Verification items for the finished model (mm, model axes). A direction names the side the tool comes from. Coordinates: 2 decimals unless noted, no trailing zeros. Loops run counter-clockwise (first coordinate to the right, second up) from the corner with the lowest first, then second, coordinate; pieces in that order, holes last. Notation, with made-up numbers: M 31,61.5 L 40,61.5 A10 cw 40,80.5 Z; hole C 58.25,23 d7. An arc over 180 degrees is marked long. Write item = value, one per line. Start each with the question number.
```python
from build123d import *

# Parameters (mm, degrees)
F3_DEPTH = 6.001
F4_R     = 1.5
F5_DEPTH = 3.5
F6_R     = 1.25
F7_DEPTH = 11.501


with BuildPart() as f1:
    # F0 (on Top) → F1 (revolve)
    with BuildSketch(Plane.XY):
        Polygon((3, -12), (3, -4.699), (1.5, -4.699), (0.23, -3.965765), (0.23, -4.295025), (-3, -6.159867), (-3, -12), align=None)
    revolve(axis=Axis((1.9254176877, 0, 0), (1, 0, 0)))

    # F2 (on face) → F3 (cut, through all)
    with BuildSketch(Plane.YZ.offset(3)):
        with BuildLine():
            ThreePointArc((11.313708499, 4), (9.0433383971, 7.8878406827), (5.5, 10.6653645039))
            Line((5.5, 10.6653645039), (5.5, 4))
            Line((5.5, 4), (11.313708499, 4))
        make_face()
        with BuildLine():
            Line((4.6723228698, -0.5), (11.9895788083, -0.5))
            ThreePointArc((11.9895788083, -0.5), (11.9973944192, -0.2500542947), (12, 0))
            ThreePointArc((12, 0), (11.9973944192, 0.2500542947), (11.9895788083, 0.5))
            Line((11.9895788083, 0.5), (4.6723228698, 0.5))
            ThreePointArc((4.6723228698, 0.5), (4.6923259779, 0.2503555818), (4.699, 0))
            ThreePointArc((4.699, 0), (4.6923259779, -0.2503555818), (4.6723228698, -0.5))
        make_face()
        with BuildLine():
            Line((-10, -0.5), (-4.6723228698, -0.5))
            ThreePointArc((-4.6723228698, -0.5), (-4.699, 0), (-4.6723228698, 0.5))
            Line((-4.6723228698, 0.5), (-10, 0.5))
            Line((-10, 0.5), (-10, -0.5))
        make_face()
        with BuildLine():
            Line((-4.6723228698, -0.5), (4.6723228698, -0.5))
            ThreePointArc((4.6723228698, -0.5), (4.6923259779, -0.2503555818), (4.699, 0))
            ThreePointArc((4.699, 0), (4.6923259779, 0.2503555818), (4.6723228698, 0.5))
            Line((4.6723228698, 0.5), (-4.6723228698, 0.5))
            ThreePointArc((-4.6723228698, 0.5), (-4.699, 0), (-4.6723228698, -0.5))
        make_face()
    extrude(amount=-F3_DEPTH, mode=Mode.SUBTRACT)

    # F4 (on face) → F5 (cut, through all)
    with BuildSketch(Plane.XY.offset(4)):
        with Locations((0, 8.5)):
            Circle(F4_R)
    extrude(amount=-F5_DEPTH, mode=Mode.SUBTRACT)

    # F6 (on face) → F7 (cut, through all)
    with BuildSketch(Plane.XY.offset(-0.5)):
        with Locations((0, 8.5)):
            Circle(F6_R)
    extrude(amount=-F7_DEPTH, mode=Mode.SUBTRACT)


solid = f1.part
```
Q1. Mould release check, pull along Y, two halves, no side actions. Record for faces 5 (the face through (0, 5.5, 7)), 6 (the face through (-0.27, 7.28, -4.97)), 7 (the face through (0, -8, -0.5)): +Y half, -Y half, draft (parallel to the pull), parting line (faces both ways), or undercut.
Q2. Sectioned sample at C-C on z = 0. Record the cut outline in (x, y).
Q3. Set-up check for faces 1 (the face through (1, 7, 4)), 2 (the face through (1.4, 8.8, -0.5)), 3 (the face through (-0.69, 0.101, 4.825)), 4 (the face through (0.43, 0.08, 4.08)): record each of +Z, -Z, +X, -X, +Y, -Y from which the full face is reachable in a straight line by a thin tool's end or side.
Q4. Sectioned sample at A-A on y = 8.5. Record the cut outline in (x, z), plus the area to 3 significant figures.
Q5. Gauge pin test, flat ends, axial feed: pin 1 (1.5 mm diameter, centred on x = 1.5, y = -4, fed in from -Z); pin 2 (1.1 mm diameter, centred on y = 0, z = 2, fed in from -X); pin 3 (3 mm diameter, centred on x = 0.5, y = 9.5, fed in from +Z); pin 4 (3 mm diameter, centred on x = 1, y = -7, fed in from -Z). Record the tip position at first contact, or that the pin passes through.
Q6. Sectioned sample at D-D on y = -9.5. Record the cut outline in (x, z).
Q7. Scan lines: L1, parallel to X at y = 8.5, z = -4.5; L2, parallel to Y at x = 1, z = 2.5; L3, parallel to Y at x = 2.75, z = -2.25. Record each from-to range of solid material in increasing order. Write a range as [from, to].
Q8. Sectioned sample at B-B on y = 0. Record the cut outline in (x, z).
Solutions:
q1.face_5 = +Y half
q1.face_6 = undercut
q1.face_7 = draft
q2.outline = M -3,-12 L 3,-12 L 3,-10 L -3,-10 Z
q3.face_1 = +Z, +X, -X, +Y
q3.face_2 = +X, -X, +Y
q3.face_3 = -X
q3.face_4 = +X
q4.outline = M -3,-8.47 L -1.25,-8.47 L -1.25,-0.5 L -3,-0.5 Z; M -3,0.5 L -1.5,0.5 L -1.5,4 L -3,4 Z; M 1.25,-8.47 L 3,-8.47 L 3,-0.5 L 1.25,-0.5 Z; M 1.5,0.5 L 3,0.5 L 3,4 L 1.5,4 Z
q4.area = 38.4 mm²
q5.pin_1 = -11.55
q5.pin_2 = through
q5.pin_3 = 4
q5.pin_4 = -10.67
q6.outline = M -3,-7.33 L 3,-7.33 L 3,-0.5 L -3,-0.5 Z; M -3,0.5 L 3,0.5 L 3,7.33 L -3,7.33 Z
q7.L1 = [-3, -1.25], [1.25, 3]
q7.L2 = [-11.74, -3.63], [3.63, 7.38], [9.62, 11.74]
q7.L3 = [-11.79, -4.13], [4.13, 11.79]
q8.outline = M -3,-12 L 3,-12 L 3,-4.7 L 1.5,-4.7 L 0.23,-3.97 L 0.23,-4.3 L -3,-6.16 Z; M -3,6.16 L 0.23,4.3 L 0.23,3.97 L 1.5,4.7 L 3,4.7 L 3,12 L -3,12 Z
